```python
from build123d import *

# Parameters (mm, degrees)
SKETCH1_W           = 26
SKETCH1_H           = 20
BOSS_EXTRUDE1_DEPTH = 18
HOLE1_D             = 4.4
HOLE2_D             = 3.33839548
HOLE3_D             = 8


with BuildPart() as part:
    # Sketch1 → Boss-Extrude1 (new body)
    with BuildSketch(Plane(origin=(-47, 0, 0), x_dir=(0, -1, 0), z_dir=(-1, 0, 0))):
        with Locations((0, 8)):
            Rectangle(SKETCH1_W, SKETCH1_H)
    extrude(amount=-BOSS_EXTRUDE1_DEPTH)

    # Hole1 (through all)
    with Locations(Plane.ZY.offset(47)):
        with Locations((8, 7)):
            Hole(HOLE1_D / 2)

    # Hole2 (through all)
    with Locations(Plane.ZY.offset(47)):
        with Locations((8, -7)):
            Hole(HOLE2_D / 2)

    # Hole3 (through all)
    with Locations(Plane(origin=(0, 0, -2), x_dir=(-1, 0, 0), z_dir=(0, 0, -1))):
        with Locations((29, 0)):
            Hole(HOLE3_D / 2)


solid = part.part
```
Source: CAD feature listing. Evaluate the final solid. Frame: model axes, mm. Round coordinates to 2 decimals unless told otherwise and drop trailing zeros. Loops run counter-clockwise (first coordinate to the right, second up) from the corner with the lowest first, then second, coordinate; pieces in that order, holes last. Notation, with made-up numbers: M 14,12.25 L 49,12.25 A20 ccw 49,26.25 Z; hole C 23.25,-36.5 d5. An arc over 180 degrees is marked long. Use a Markdown table: item, result. Add a question column.
1. Cut plane D-D, the plane x = -44.75. Output: boundary loops of the cut face in (y, z).
2. Ray query, line 1 along Y through (x, z) = (-33.5, 8); line 2 along Y through (x, z) = (-36, 7); line 3 along Z through (x, y) = (-37.75, 5.75). Return the intervals inside material, ascending. Write a range as [from, to].
3. Cut plane B-B, the plane x = -31. Output: boundary loops of the cut face in (y, z), and give its area (3 significant figures).
4. Pull-direction query (Y, two-part tool) for faces 1 (the cylindrical face through (-37.87, -7.64, 6.46)), 2 (the flat face through (-38, -13, 8)), 3 (the flat face through (-38, 0, -2)); classes: +Y half, -Y half, draft (parallel to the pull), parting line (faces both ways), or undercut.
5. Cut plane C-C, the plane y = 7. Output: boundary loops of the cut face in (x, z), and give its area (3 significant figures).
6. Cut plane A-A, the plane z = 8. Output: boundary loops of the cut face in (x, y).
Solution:
| question | item | result |
|---|---|---|
| 1 | outline | M -13,-2 L 13,-2 L 13,18 L -13,18 Z; hole C -7,8 d3.34; hole C 7,8 d4.4 |
| 2 | line 1 | y = [-13, -8.67], [-5.33, 4.8], [9.2, 13] |
| 2 | line 2 | y = [-13, -8.34], [-5.66, 5.04], [8.96, 13] |
| 2 | line 3 | z = [-2, 6.19], [9.81, 18] |
| 3 | outline | M -13,-2 L -3.46,-2 L -3.46,18 L -13,18 Z; M 3.46,-2 L 13,-2 L 13,18 L 3.46,18 Z; hole C -7,8 d3.34; hole C 7,8 d4.4 |
| 3 | area | 357 mm2 |
| 4 | face 1 | undercut |
| 4 | face 2 | -Y half |
| 4 | face 3 | draft |
| 5 | outline | M -47,-2 L -29,-2 L -29,5.8 L -47,5.8 Z; M -47,10.2 L -29,10.2 L -29,18 L -47,18 Z |
| 5 | area | 281 mm2 |
| 6 | outline | M -47,-13 L -29,-13 L -29,-8.67 L -47,-8.67 Z; M -47,-5.33 L -29,-5.33 L -29,-4 A4 cw -29,4 L -29,4.8 L -47,4.8 Z; M -47,9.2 L -29,9.2 L -29,13 L -47,13 Z |
